Can you work these out from the model? Positions are in its coordinate system, mm. Face numbers are marked on the shaded views. A direction names the side the tool comes from. Coordinates: 2 decimals unless noted, no trailing zeros. Write each loop counter-clockwise with the first axis right and the second up, starting at its lowest first coordinate (ties: lowest second). Pieces come first, ordered by that corner, then holes. Notation, with made-up numbers: (8, 67) - (67, 67) arc R21 ccw to (67, 71) - close; hole circle Ø2 at (42.25, -7.5). An arc over 180 degrees is marked (long way). Write each question's results on one line, items separated by ' | '. Start each with the question number.
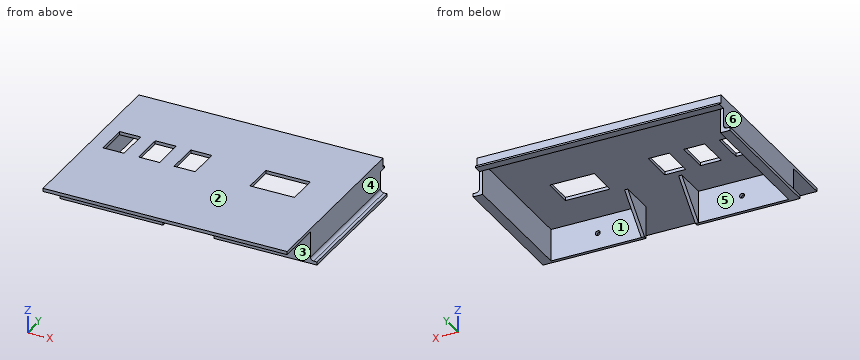
```python
from build123d import *

# Parameters (mm, degrees)
SKETCH1_W            = 151
SKETCH1_H            = 115
BOSS_EXTRUDE1_DEPTH  = 2
SKETCH2_W            = 13
SKETCH2_H            = 20
CUT_EXTRUDE1_DEPTH   = 2
SKETCH3_W            = 27.5
SKETCH3_H            = 19
CUT_EXTRUDE2_DEPTH   = 2
SKETCH4_W            = 151
SKETCH4_H            = 3
BOSS_EXTRUDE2_DEPTH  = 4
SKETCH6_W            = 151
SKETCH6_H            = 5
BOSS_EXTRUDE3_DEPTH  = 1
FILLET1_R            = 1
SKETCH7_W            = 2
SKETCH7_H            = 84
BOSS_EXTRUDE4_DEPTH  = 10
SKETCH8_W            = 27.5
SKETCH8_H            = 19
SKETCH8_W_2          = 13
SKETCH8_H_2          = 20
CUT_EXTRUDE3_DEPTH   = 10
SKETCH9_W            = 126.512620881
SKETCH9_H            = 26.913833817
BOSS_EXTRUDE5_DEPTH  = 2
SKETCH10_W           = 2
SKETCH10_H           = 84
BOSS_EXTRUDE6_DEPTH  = 8
SKETCH12_W           = 6
SKETCH12_H           = 84
BOSS_EXTRUDE7_DEPTH  = 2
FILLET2_R            = 2
FILLET3_R            = 2
SKETCH14_W           = 57.787784132
SKETCH14_H           = 20
SKETCH14_W_2         = 59.787784131
BOSS_EXTRUDE8_DEPTH  = 2
SKETCH15_R           = 1.5
CUT_EXTRUDE4_DEPTH   = 2
BOSS_EXTRUDE9_DEPTH  = 2
BOSS_EXTRUDE10_DEPTH = 2


with BuildPart() as part:
    # Sketch1 → Boss-Extrude1 (new body)
    with BuildSketch(Plane.XY):
        with Locations((1.428458571, -7.256892256)):
            Rectangle(SKETCH1_W, SKETCH1_H)
    extrude(amount=BOSS_EXTRUDE1_DEPTH)

    # Sketch2 → Cut-Extrude1 (cut)
    with BuildSketch(Plane.XY.offset(2)):
        with Locations((-58.571541429, -29.756892256)):
            Rectangle(SKETCH2_W, SKETCH2_H)
        with Locations((-36.571541429, -29.756892256)):
            Rectangle(SKETCH2_W, SKETCH2_H)
        with Locations((-14.571541429, -29.756892256)):
            Rectangle(SKETCH2_W, SKETCH2_H)
    extrude(amount=-CUT_EXTRUDE1_DEPTH, mode=Mode.SUBTRACT)

    # Sketch3 → Cut-Extrude2 (cut)
    with BuildSketch(Plane.XY.offset(2)):
        with Locations((39.228458571, -29.756892256)):
            Rectangle(SKETCH3_W, SKETCH3_H)
    extrude(amount=-CUT_EXTRUDE2_DEPTH, mode=Mode.SUBTRACT)

    # Sketch4 → Boss-Extrude2 (add)
    with BuildSketch(Plane(origin=(0, 0, 0), x_dir=(-1, 0, 0), z_dir=(0, 0, -1))):
        with Locations((-1.428458571, 48.743107744)):
            Rectangle(SKETCH4_W, SKETCH4_H)
    extrude(amount=BOSS_EXTRUDE2_DEPTH)

    # Sketch6 → Boss-Extrude3 (add)
    with BuildSketch(Plane(origin=(0, 0, -4), x_dir=(-1, 0, 0), z_dir=(0, 0, -1))):
        with Locations((-1.428458571, 49.743107744)):
            Rectangle(SKETCH6_W, SKETCH6_H)
    extrude(amount=BOSS_EXTRUDE3_DEPTH)

    # Fillet1
    fillet1_edges = [part.edges().sort_by_distance(p)[0] for p in [
        (1.428458571, 50.243107744, -4),
    ]]
    fillet(fillet1_edges, radius=FILLET1_R)

    # Sketch7 → Boss-Extrude4 (add)
    with BuildSketch(Plane(origin=(0, 0, 0), x_dir=(-1, 0, 0), z_dir=(0, 0, -1))):
        with Locations((-75.928458571, 5.243107744)):
            Rectangle(SKETCH7_W, SKETCH7_H)
        with Locations((73.071541429, 5.243107744)):
            Rectangle(SKETCH7_W, SKETCH7_H)
    extrude(amount=BOSS_EXTRUDE4_DEPTH)

    # Sketch8 → Cut-Extrude3 (cut)
    with BuildSketch(Plane(origin=(0, 0, 0), x_dir=(-1, 0, 0), z_dir=(0, 0, -1))):
        with Locations((-39.604851179, -0.756892256)):
            Rectangle(SKETCH8_W, SKETCH8_H)
        with Locations((14.571541429, -0.256892256)):
            Rectangle(SKETCH8_W_2, SKETCH8_H_2)
        with Locations((36.571541429, -0.256892256)):
            Rectangle(SKETCH8_W_2, SKETCH8_H_2)
        with Locations((58.571541429, -0.256892256)):
            Rectangle(SKETCH8_W_2, SKETCH8_H_2)
    extrude(amount=-CUT_EXTRUDE3_DEPTH, mode=Mode.SUBTRACT)

    # Sketch9 → Boss-Extrude5 (add)
    with BuildSketch(Plane(origin=(0, 0, 0), x_dir=(-1, 0, 0), z_dir=(0, 0, -1))):
        with Locations((5.18783125, -30.15024479)):
            Rectangle(SKETCH9_W, SKETCH9_H)
    extrude(amount=-BOSS_EXTRUDE5_DEPTH)

    # Sketch10 → Boss-Extrude6 (add)
    with BuildSketch(Plane(origin=(0, 0, -10), x_dir=(-1, 0, 0), z_dir=(0, 0, -1))):
        with Locations((-75.928458571, 5.243107744)):
            Rectangle(SKETCH10_W, SKETCH10_H)
        with Locations((73.071541429, 5.243107744)):
            Rectangle(SKETCH10_W, SKETCH10_H)
    extrude(amount=BOSS_EXTRUDE6_DEPTH)

    # Sketch12 → Boss-Extrude7 (add)
    with BuildSketch(Plane(origin=(0, 0, -18), x_dir=(-1, 0, 0), z_dir=(0, 0, -1))):
        with Locations((-77.928458571, 5.243107744)):
            Rectangle(SKETCH12_W, SKETCH12_H)
        with Locations((75.071541429, 5.243107744)):
            Rectangle(SKETCH12_W, SKETCH12_H)
    extrude(amount=BOSS_EXTRUDE7_DEPTH)

    # Fillet2
    fillet2_edges = [part.edges().sort_by_distance(p)[0] for p in [
        (76.928458571, 5.243107744, -18),
    ]]
    fillet(fillet2_edges, radius=FILLET2_R)

    # Fillet3
    fillet3_edges = [part.edges().sort_by_distance(p)[0] for p in [
        (-74.071541429, 5.243107744, -18),
    ]]
    fillet(fillet3_edges, radius=FILLET3_R)

    # Sketch14 → Boss-Extrude8 (add)
    with BuildSketch(Plane(origin=(0, -36.756892256, 0), x_dir=(-1, 0, 0), z_dir=(0, -1, 0))):
        with Locations((-46.034566505, 10)):
            Rectangle(SKETCH14_W, SKETCH14_H)
        with Locations((44.177649364, 10)):
            Rectangle(SKETCH14_W_2, SKETCH14_H)
    extrude(amount=-BOSS_EXTRUDE8_DEPTH)

    # Sketch15 → Cut-Extrude4 (cut)
    with BuildSketch(Plane(origin=(0, -34.756892256, 0), x_dir=(1, 0, 0), z_dir=(0, 1, 0))):
        with Locations((46.034566505, 10)):
            Circle(SKETCH15_R)
        with Locations((-43.177649364, 10)):
            Circle(SKETCH15_R)
    extrude(amount=-CUT_EXTRUDE4_DEPTH, mode=Mode.SUBTRACT)

    # Sketch16 → Boss-Extrude9 (add)
    with BuildSketch(Plane.ZY.offset(-17.140674439)):
        Polygon((0, -34.756892256), (-20, -34.756892256), (0, -14.756892256), align=None)
    extrude(amount=-BOSS_EXTRUDE9_DEPTH)

    # Sketch18 → Boss-Extrude10 (add)
    with BuildSketch(Plane(origin=(-14.283757298, 0, 0), x_dir=(0, 0, -1), z_dir=(1, 0, 0))):
        Polygon((0, -34.756892256), (20, -34.756892256), (0, -14.756892256), align=None)
    extrude(amount=-BOSS_EXTRUDE10_DEPTH)


solid = part.part
```
Q1. If we section it at B-B (z = -14): Please give me the cut outline in (x, y).
Q2. If we section it at D-D (y = 39): Please give me the cut outline in (x, z), then the cut area to 3 significant figures.
Q3. I need wall thicknesses on line 1 along X through (y, z) = (-36.05, -10); line 2 along X through (y, z) = (40, -6.75); line 3 along Z through (x, y) = (50, -19). Which ranges of each line are inside material? Lowest first, please. Write a range as from..to.
Q4. I'm going to push flat-ended pins straight in: pin 1 Ø0.6 at (x, z) = (-57.5, 1) entering from +Y; pin 2 Ø1.1 at (x, y) = (-33, 51.5) entering from +Z; pin 3 Ø4 at (y, z) = (-33, -8.5) entering from -X; pin 4 Ø10 at (x, z) = (25, -4.5) entering from -Y. Where does each tip first touch, or does it pass through?
Q5. If we section it at C-C (y = -5.5): Count the separate pieces of the cut face and the enclosed holes in it, then the cut area to 3 significant figures.
Q6. Thinking about a two-plate mould opening in Y: for the marked faces 1, 2 and 3, which applies, pulls with the +Y half, pulls with the -Y half, needs draft (parallel to the pull), parting line crosses it, or undercut?
Q7. For the marked faces 4, 5 and 6, which set-ups out of +Z, -Z, +X, -X, +Y, -Y let a thin tool reach every point of the face, with its end or its side?
Q8. If we section it at A-A (x = -34): Please give me the cut outline in (y, z), then the cut area to 3 significant figures.
Answer list:
1) outline: (-74.07, -36.76) - (-14.28, -36.76) - (-14.28, -28.76) - (-16.28, -28.76) - (-16.28, -34.76) - (-72.07, -34.76) - (-72.07, 47.24) - (-74.07, 47.24) - close; (17.14, -36.76) - (76.93, -36.76) - (76.93, 47.24) - (74.93, 47.24) - (74.93, -34.76) - (19.14, -34.76) - (19.14, -28.76) - (17.14, -28.76) - close
2) outline: (-78.07, -20) - (-72.07, -20) - (-72.07, 0) - (74.93, 0) - (74.93, -20) - (80.93, -20) - (80.93, -18) - (78.93, -18) arc R2 cw to (76.93, -16) - (76.93, 2) - (-74.07, 2) - (-74.07, -16) arc R2 cw to (-76.07, -18) - (-78.07, -18) - close | area: 400 mm2
3) line 1: x = -74.07..-44.68, -41.68..-14.28, 17.14..44.53, 47.53..76.93 | line 2: x = -74.07..-72.07, 74.93..76.93 | line 3: z = 0..2
4) pin 1: stops at y = 50.24 | pin 2: stops at z = -3.96 | pin 3: stops at x = -74.07 | pin 4: stops at y = -64.76
5) separate pieces: 5 | enclosed holes: 0 | area: 267 mm2
6) face 1: undercut | face 2: needs draft | face 3: pulls with the -Y half
7) face 4: +Z, +X, +Y, -Y | face 5: -Z | face 6: +Z, -X, +Y, -Y
8) outline: (-64.76, 0) - (-36.76, 0) - (-36.76, -20) - (-34.76, -20) - (-34.76, 0) - (-10.26, 0) - (-10.26, 2) - (-64.76, 2) - close; (9.74, 0) - (47.24, 0) - (47.24, -5) - (52.24, -5) - (52.24, -4) - (51.24, -4) arc R1 cw to (50.24, -3) - (50.24, 2) - (9.74, 2) - close | area: 247 mm2
